Geometry check sheet. Reference: the model listing, model coordinates, mm. Round coordinates to 2 decimals unless told otherwise and drop trailing zeros. Loops run counter-clockwise (first coordinate to the right, second up) from the corner with the lowest first, then second, coordinate; pieces in that order, holes last. Notation, with made-up numbers: (34.5, 60.25) - (76.5, 60.25) arc R26 cw to (76.5, 92.25) - close; hole circle Ø1 at (28.25, 81). An arc over 180 degrees is marked (long way). Answer as CSV lines item,"result". Start each with the question number.
1) Depth check by flat-ended pin: P1, Ø6, axis at y = 19.5, z = 518.5, coming from the -X side; P2, Ø25, axis at x = -50.5, y = -3.5, coming from the -Z side; P3, Ø9.5, axis at x = -52, y = 4, coming from the +Z side; P4, Ø1.5, axis at x = -37.5, z = 1005, coming from the -Y side. Enter the tip coordinate at first touch or a pass-through.
2) Cross-section at B-B on x = -54. Record the boundary of the cut face in (y, z).
3) Thickness scan on line 1 along Z through (x, y) = (58, -4); line 2 along X through (y, z) = (-28.5, 1190). Record the ranges inside material, lowest first.
4) Cross-section at C-C on z = 325.5. Record the boundary of the cut face in (x, y).
5) Cross-section at A-A on y = -13. Record the boundary of the cut face in (x, z), and give its area (3 significant figures).
from build123d import *

# Parameters (mm, degrees)
F0_W     = 73
F0_H     = 73
F1_DEPTH = 1555
F2_W     = 65
F2_H     = 31
F3_DEPTH = 31
F4_W     = 67
F4_H     = 31
F5_DEPTH = 57


with BuildPart() as f1:
    # F0 (on Top) → F1 (new body)
    with BuildSketch(Plane.XY):
        Rectangle(F0_W, F0_H)
    extrude(amount=F1_DEPTH)

    # F2 (on face) → F3 (join)
    with BuildSketch(Plane(origin=(-36.5, 0, 0), x_dir=(0, -1, 0), z_dir=(-1, 0, 0))):
        with Locations((0, 60.5)):
            Rectangle(F2_W, F2_H)
    extrude(amount=F3_DEPTH)

    # F4 (on face) → F5 (join)
    with BuildSketch(Plane.YZ.offset(36.5)):
        with Locations((0, 60.5)):
            Rectangle(F4_W, F4_H)
    extrude(amount=F5_DEPTH)


solid = f1.part
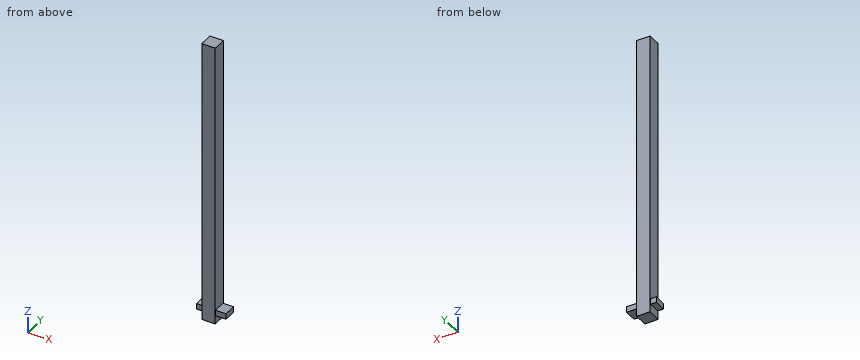
Answer block:
1,P1,"stops at x = -36.5"
1,P2,"stops at z = 45"
1,P3,"stops at z = 76"
1,P4,"passes through"
2,outline,"(-32.5, 45) - (32.5, 45) - (32.5, 76) - (-32.5, 76) - close"
3,line 1,"z = 45 to 76"
3,line 2,"x = -36.5 to 36.5"
4,outline,"(-36.5, -36.5) - (36.5, -36.5) - (36.5, 36.5) - (-36.5, 36.5) - close"
5,outline,"(-67.5, 45) - (-36.5, 45) - (-36.5, 0) - (36.5, 0) - (36.5, 45) - (93.5, 45) - (93.5, 76) - (36.5, 76) - (36.5, 1555) - (-36.5, 1555) - (-36.5, 76) - (-67.5, 76) - close"
5,area,"116,000 mm^2"
